Build history of the part. All positions in model axes, mm. Give positions to 0.01 mm unless a question says otherwise; leave off trailing zeros. Order: outer loops, then holes, each group sorted by start corner. A loop starts at its lowest first (then second) coordinate and runs counter-clockwise, first axis right, second up. Notation, with made-up numbers: (67.25, 79) - (104.25, 79) arc R17 cw to (104.25, 107) - close; hole circle Ø9 at (9.25, -12.5). An arc over 180 degrees is marked (long way). Write each question's results on one line, items separated by ' | '. Start each with the question number.
1) Cut at B-B on y = 311.5. List the corners of the cut face in (x, z), plus the area to 3 significant figures.
2) Drill centre lines: line 1 along Y through (x, z) = (7, 448); line 2 along Y through (x, z) = (208, 449.5); line 3 along Z through (x, y) = (226, 180.5). Where is each one in solid material? Low to high. Write a range as from..to.
3) Cut at A-A on x = -177. List the corners of the cut face in (y, z), plus the area to 3 significant figures.
4) Cut at C-C on z = 429.5. List the corners of the cut face in (x, y), plus the area to 3 significant figures.
5) Drop flat-ended pins along their axis: pin 1 Ø8 at (x, y) = (135.5, 209) entering from +Z; pin 2 Ø6 at (x, y) = (23.5, 315) entering from +Z; pin 3 Ø10 at (x, y) = (-234.5, 108) entering from +Z; pin 4 Ø11.5 at (y, z) = (383.12, 448.8) entering from -X. Give the stop position or say it passes through.
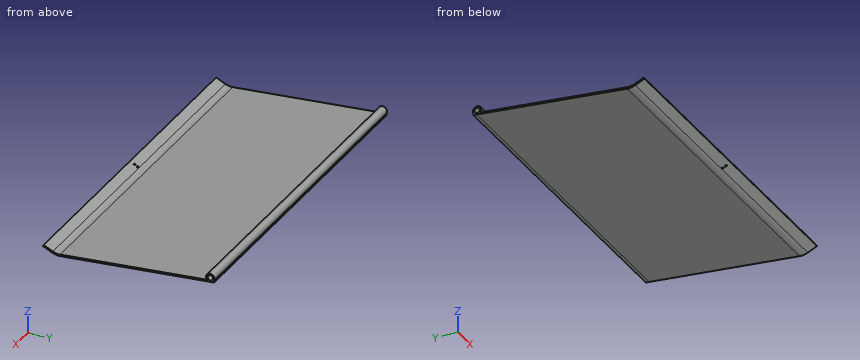
from build123d import *

# Parameters (mm, degrees)
MAIN_DEPTH       = 300
SCREW_HOLE_REACH = 387.023
SKETCH3_R        = 1.75


with BuildPart() as part:
    # Sketch2 → Main (new, symmetric)
    # profile 1 of 4: a face of its own
    with BuildSketch(Plane(origin=(0, 0, 0), x_dir=(0, 0, -1), z_dir=(1, 0, 0))):
        with BuildLine():
            ThreePointArc((-444.632221398, 389.90913895), (-442.099910912, 387.426906528), (-440.895406833, 384.091753741))
            Line((-440.895406833, 384.091753741), (-441.695942664, 390.611594874))
            Line((-441.695942664, 390.611594874), (-444.673581118, 390.245986843))
            Line((-444.673581118, 390.245986843), (-444.632221398, 389.90913895))
        make_face()
    # profile 2 of 4: a face of its own
    with BuildSketch(Plane(origin=(0, 0, 0), x_dir=(0, 0, -1), z_dir=(1, 0, 0))):
        with BuildLine():
            Line((-418.365390033, 66.409688449), (-415.614602943, 65.212537504))
            Line((-415.614602943, 65.212537504), (-408.006110333, 82.695164353))
            ThreePointArc((-408.006110333, 82.695164353), (-405.861496509, 90.229320908), (-405.775405247, 98.062294273))
            Line((-405.775405247, 98.062294273), (-440.895406833, 384.091753741))
            ThreePointArc((-440.895406833, 384.091753741), (-440.850878518, 383.607155927), (-440.836017267, 383.120743597))
            ThreePointArc((-440.836017267, 383.120743597), (-441.427429555, 380.10834645), (-443.113869014, 377.543151133))
            Line((-443.113869014, 377.543151133), (-408.753043702, 97.696686242))
            ThreePointArc((-408.753043702, 97.696686242), (-408.83037992, 90.66028644), (-410.756897423, 83.892315298))
            Line((-410.756897423, 83.892315298), (-418.365390033, 66.409688449))
        make_face()
    # profile 3 of 4: a face of its own
    with BuildSketch(Plane(origin=(0, 0, 0), x_dir=(0, 0, -1), z_dir=(1, 0, 0))):
        with BuildLine():
            ThreePointArc((-440.836017267, 383.120743597), (-440.850878518, 383.607155927), (-440.895406833, 384.091753741))
            ThreePointArc((-440.895406833, 384.091753741), (-442.099910912, 387.426906528), (-444.632221398, 389.90913895))
            Line((-444.632221398, 389.90913895), (-443.873045205, 383.726145039))
            Line((-443.873045205, 383.726145039), (-443.113869014, 377.543151133))
            ThreePointArc((-443.113869014, 377.543151133), (-441.427429555, 380.10834645), (-440.836017267, 383.120743597))
        make_face()
    # profile 4 of 4: a face of its own
    with BuildSketch(Plane(origin=(0, 0, 0), x_dir=(0, 0, -1), z_dir=(1, 0, 0))):
        with BuildLine():
            Line((-443.873045205, 383.726145039), (-444.632221398, 389.90913895))
            ThreePointArc((-444.632221398, 389.90913895), (-456.711881838, 382.149734123), (-443.113869014, 377.543151133))
            Line((-443.113869014, 377.543151133), (-443.873045205, 383.726145039))
        make_face()
        with BuildLine():
            ThreePointArc((-443.836017267, 383.120743597), (-453.762005696, 382.817477223), (-443.873045205, 383.726145039))
            ThreePointArc((-443.873045205, 383.726145039), (-443.845282893, 383.424009971), (-443.836017267, 383.120743597))
        make_face(mode=Mode.SUBTRACT)
    extrude(amount=MAIN_DEPTH, both=True)

    # Sketch3 → Screw Hole (cut, up to next)
    with BuildSketch(Plane(origin=(0, 163.655393922, 376.043761949), x_dir=(1, 0, 0), z_dir=(0, 0.3990503148824781, 0.9169290300738631)), mode=Mode.PRIVATE) as screw_hole_sk1:
        with Locations(Location((0, -96.522619686, 0), (0, 0, 270))):
            Circle(SKETCH3_R)
    screw_hole_tool1 = extrude(screw_hole_sk1.sketch, amount=-SCREW_HOLE_REACH, mode=Mode.PRIVATE) & part.part
    # Sketch3 → Screw Hole (cut, up to next)
    with BuildSketch(Plane(origin=(0, 163.655393922, 376.043761949), x_dir=(1, 0, 0), z_dir=(0, 0.3990503148824781, 0.9169290300738631)), mode=Mode.PRIVATE) as screw_hole_sk2:
        with Locations(Location((0, -89.666587201, 0), (0, 0, 270))):
            Circle(SKETCH3_R)
    screw_hole_tool2 = extrude(screw_hole_sk2.sketch, amount=-SCREW_HOLE_REACH, mode=Mode.PRIVATE) & part.part
    add(screw_hole_tool1.solids().sort_by_distance((0, 75.151002, 414.561144))[0], mode=Mode.SUBTRACT)
    add(screw_hole_tool2.solids().sort_by_distance((0, 81.437497, 411.825242))[0], mode=Mode.SUBTRACT)


solid = part.part
Results:
1) outline: (-300, 431.98) - (300, 431.98) - (300, 435) - (-300, 435) - close | area: 1,810 mm^2
2) line 1: 375.19..378.22, 388.02..391.05 | line 2: 375.18..378.2, 388.04..391.06 | line 3: 415.9..418.92
3) outline: (65.21, 415.61) - (82.7, 408.01) arc R29.5 ccw to (98.06, 405.78) - (390.61, 441.7) - (390.25, 444.67) - (389.91, 444.63) arc R7.97 ccw (long way) to (377.54, 443.11) - (97.7, 408.75) arc R26.5 cw to (83.89, 410.76) - (66.41, 418.37) - close; hole circle Ø9.94 at (383.12, 448.8) | area: 1,080 mm^2
4) outline: (-300, 266.67) - (300, 266.67) - (300, 291.28) - (-300, 291.28) - close | area: 14,800 mm^2
5) pin 1: z = 422.91 | pin 2: z = 435.8 | pin 3: z = 410.63 | pin 4: x = -300
